Geometry check sheet. Reference: drawing and pictorial views, mm from the part's lowest x, y, z. A direction names the side the tool comes from. Coordinates: 2 decimals unless noted, no trailing zeros. Write each loop counter-clockwise with the first axis right and the second up, starting at its lowest first coordinate (ties: lowest second). Pieces come first, ordered by that corner, then holes. Notation, with made-up numbers: (73.5, -19) -> (110.5, -19) arc R21 ccw to (110.5, -10) -> close; hole circle Ø3 at (-9, -35.5). An arc over 180 degrees is marked (long way). Put each result on its own line as item: value.
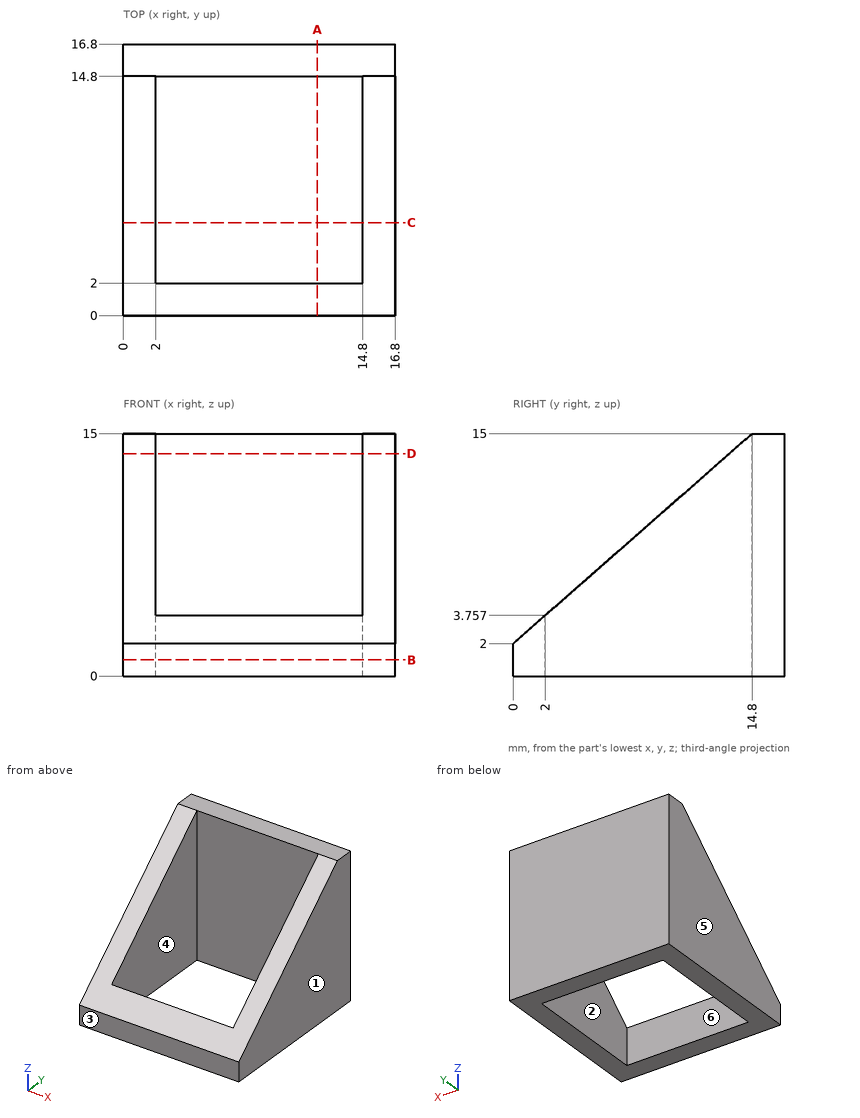
Q1. Mould release check, pull along Y, two halves, no side actions. Record for the marked faces 1, 2, 3 and 4: released by +Y, released by -Y, zero draft, split by the parting line, or undercut.
Recorded:
face 1: zero draft
face 2: undercut
face 3: released by -Y
face 4: undercut
Q2. Cross-section at A-A (x = 12). Record the cut outline in (y, z).
Recorded:
outline: (0, 0) -> (2, 0) -> (2, 3.76) -> (0, 2) -> close; (14.8, 0) -> (16.8, 0) -> (16.8, 15) -> (14.8, 15) -> close
Q3. Cross-section at D-D (z = 13.75). Record the cut outline in (x, y), plus the area to 3 significant figures.
Recorded:
outline: (0, 13.38) -> (2, 13.38) -> (2, 14.8) -> (14.8, 14.8) -> (14.8, 13.38) -> (16.8, 13.38) -> (16.8, 16.8) -> (0, 16.8) -> close
area: 39.3 mm2
Q4. Cross-section at B-B (z = 1). Record the cut outline in (x, y), plus the area to 3 significant figures.
Recorded:
outline: (0, 0) -> (16.8, 0) -> (16.8, 16.8) -> (0, 16.8) -> close; hole (2, 2) -> (14.8, 2) -> (14.8, 14.8) -> (2, 14.8) -> close
area: 118 mm2
Q5. Tool access check on the marked faces 5 and 6. Record the directions out of +Z, -Z, +X, -X, +Y, -Y that give a thin tool (end or side, any length) a straight path to the whole face; none if there is none.
Recorded:
face 5: +Z, -Z, -X, +Y, -Y
face 6: +Z, -Z
Q6. Material ranges on line 1 along X through (y, z) = (6.5, 1.5); line 2 along Y through (x, z) = (5.75, 12), recorded low to high.
Recorded:
line 1: x = 0 to 2, 14.8 to 16.8
line 2: y = 14.8 to 16.8
Q7. Cross-section at C-C (y = 5.75). Record the cut outline in (x, z), plus the area to 3 significant figures.
Recorded:
outline: (0, 0) -> (2, 0) -> (2, 7.05) -> (0, 7.05) -> close; (14.8, 0) -> (16.8, 0) -> (16.8, 7.05) -> (14.8, 7.05) -> close
area: 28.2 mm2
